Can you work these out from the model? Positions are in its coordinate system, mm. Face numbers are marked on the shaded views. A direction names the side the tool comes from. Give positions to 0.01 mm unless a question says otherwise; leave off trailing zeros. Loops run counter-clockwise (first coordinate to the right, second up) from the corner with the lowest first, then second, coordinate; pieces in that order, holes last. Notation, with made-up numbers: (-34, -1) - (-23, -1) arc R6 ccw to (-23, 8) - close; hole circle Ø2 at (5, 58.25). An arc over 180 degrees is marked (long way). Write item = value, one per line.
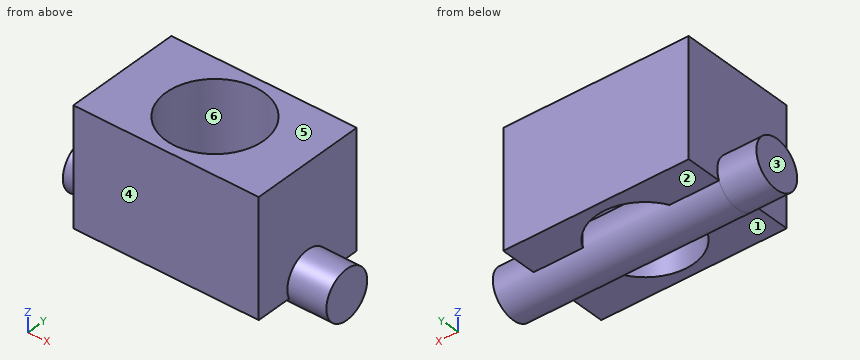
from build123d import *

# Parameters (mm, degrees)
SKETCH1_W                = 95
SKETCH1_H                = 60
SKETCH1_R                = 25
BOSS_EXTRUDE1_DEPTH      = 60
SKETCH2_R                = 12.5
BOSS_EXTRUDE2_DEPTH      = 20
BOSS_EXTRUDE2_DEPTH_BACK = 115


with BuildPart() as part:
    # Sketch1 → Boss-Extrude1 (new body)
    with BuildSketch(Plane.XY):
        with Locations((47.5, 30)):
            Rectangle(SKETCH1_W, SKETCH1_H)
        with Locations((47.5, 30)):
            Circle(SKETCH1_R, mode=Mode.SUBTRACT)
    extrude(amount=BOSS_EXTRUDE1_DEPTH)

    # Sketch2 → Boss-Extrude2 (add, two sides)
    with BuildSketch(Plane.ZY) as boss_extrude2_sk:
        with Locations((5, 30)):
            Circle(SKETCH2_R)
    extrude(amount=BOSS_EXTRUDE2_DEPTH)
    extrude(boss_extrude2_sk.sketch, amount=-BOSS_EXTRUDE2_DEPTH_BACK)


solid = part.part
Q1. I need wall thicknesses on L1, parallel to X at y = 30, z = 19; L2, parallel to Y at x = 47.5, z = 40; L3, parallel to Z at x = 78.5, y = 43.5. Which ranges of each line are inside material? Lowest first, please.
Output:
L1 = 0 to 22.5, 72.5 to 95
L2 = 0 to 5, 55 to 60
L3 = 0 to 60
Q2. We'd pull the mould along Y, two halves only. Please class the marked faces 4, 5 and 6: released by +Y, released by -Y, zero draft, split by the parting line, or undercut.
Output:
face_4 = released by -Y
face_5 = zero draft
face_6 = undercut
Q3. For pin 1 (5 mm diameter, centred on x = 63, y = 26, fed in from -Z); pin 2 (18 mm diameter, centred on y = 36.5, z = 41, fed in from +X); pin 3 (10 mm diameter, centred on x = 44.5, y = 51.5, fed in from -Z), each with a flat end and sliding along its axis, tell me the tip position at first contact or that it passes through.
Output:
pin_1 = -7.41
pin_2 = 95
pin_3 = 0
Q4. Imagine slicing it at D-D, the plane x = 88. Write out the boundary of the cut face in (y, z), then the cut area to 3 significant figures.
Output:
outline = (0, 0) - (18.54, 0) arc R12.5 ccw to (41.46, 0) - (60, 0) - (60, 60) - (0, 60) - close
area = 3,720 mm2
Q5. Which directions (+Z, -Z, +X, -X, +Y, -Y) give clear straight access to the entire face, cutting with the end or side of a thin tool? Please do the marked faces 1, 2 and 3.
Output:
face_1 = -Z, +X, -X, -Y
face_2 = -Z, +X, -X, +Y
face_3 = +Z, -Z, -X, +Y, -Y
Q6. Imagine slicing it at C-C, the plane z = 43. Write out the boundary of the cut face in (x, y).
Output:
outline = (0, 0) - (95, 0) - (95, 60) - (0, 60) - close; hole circle Ø50 at (47.5, 30)
Q7. Imagine slicing it at A-A, the plane x = 47.5. Write out the boundary of the cut face in (y, z).
Output:
outline = (0, 0) - (5, 0) - (5, 60) - (0, 60) - close; circle Ø25 at (30, 5); (55, 0) - (60, 0) - (60, 60) - (55, 60) - close
Q8. Imagine slicing it at B-B, the plane y = 12. Write out the boundary of the cut face in (x, z).
Output:
outline = (0, 0) - (30.15, 0) - (30.15, 60) - (0, 60) - close; (64.85, 0) - (95, 0) - (95, 60) - (64.85, 60) - close
